Read the model definition and answer for the solid it produces. Units are mm, in the model's axes. Face numbers are marked on the shaded views. A direction names the side the tool comes from. Coordinates: 2 decimals unless noted, no trailing zeros. Write each loop counter-clockwise with the first axis right and the second up, starting at its lowest first coordinate (ties: lowest second). Pieces come first, ordered by that corner, then holes.
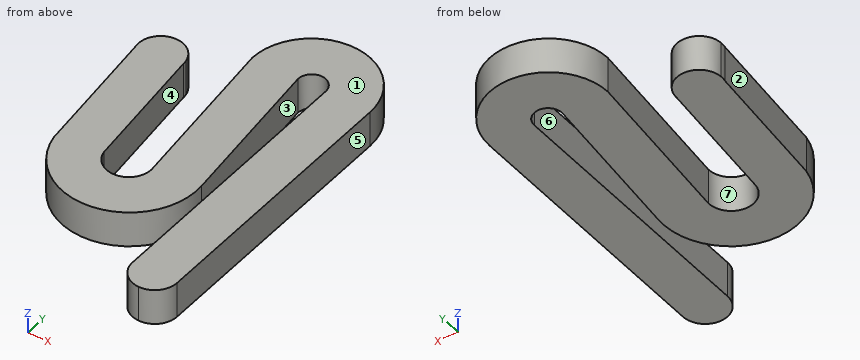
from build123d import *

# Parameters (mm, degrees)
F1_DEPTH = 5.08


with BuildPart() as f1:
    # F0 (on Top) → F1 (new body)
    with BuildSketch(Plane.XY):
        with BuildLine():
            Line((0.549417, 29.093022), (0.549417, -9.006978))
            ThreePointArc((0.549417, -9.006978), (1.479353, -11.252042), (3.724417, -12.181978))
            ThreePointArc((3.724417, -12.181978), (5.969481, -11.252042), (6.899417, -9.006978))
            Line((6.899417, -9.006978), (6.899417, 29.093022))
            ThreePointArc((6.899417, 29.093022), (-1.509537, 37.488393), (-9.891303, 29.065877))
            Line((-9.891303, 29.065877), (-7.490417, 5.875438))
            ThreePointArc((-7.490417, 5.875438), (-10.365969, 2.64314), (-13.81069, 5.260477))
            Line((-13.81069, 5.260477), (-15.701351, 23.522593))
            Line((-15.701351, 23.522593), (-15.762292, 24.111232))
            ThreePointArc((-15.762292, 24.111232), (-19.158057, 26.675151), (-22.092695, 23.594112))
            Line((-22.092695, 23.594112), (-22.003429, 22.731883))
            Line((-22.003429, 22.731883), (-20.061784, 3.977299))
            ThreePointArc((-20.061784, 3.977299), (-9.191107, -3.629406), (-1.073799, 6.865493))
            Line((-1.073799, 6.865493), (-3.372185, 29.065877))
            ThreePointArc((-3.372185, 29.065877), (-1.425051, 31.05387), (0.549417, 29.093022))
        make_face()
        with BuildLine():
            ThreePointArc((-22.092695, 23.594112), (-22.077424, 23.159958), (-22.003429, 22.731883))
            Line((-22.003429, 22.731883), (-22.092695, 23.594112))
        make_face()
        with BuildLine():
            ThreePointArc((-15.701351, 23.522593), (-15.718171, 23.818326), (-15.762292, 24.111232))
            Line((-15.762292, 24.111232), (-15.701351, 23.522593))
        make_face()
    extrude(amount=F1_DEPTH)


solid = f1.part
Item 1: For the marked faces 5, 6 and 7, determine the directions among +Z, -Z, +X, -X, +Y, -Y from which every point of the face is accessible in a straight line to the end or side of a thin tool.
Item 2: The part is cut by section B-B (x = -2.5). Give the vertices of the cut face in (y, z).
Item 3: Determine the mould class of the marked faces 1, 2, 3 and 4 for opening direction Y: +Y half, -Y half, draft (parallel to the pull), parting line (faces both ways), or undercut.
Item 4: Given pin 1 (1 mm diameter, centred on x = -4, z = 3, fed in from +Y), flat-ended and moving along its own axis, determine where the tip first touches the part or whether it passes through.
Item 5: The part is cut by section D-D (y = 13.5). Give the vertices of the cut face in (x, z).
Item 6: Find the intervals of material crossed by probe 1 along X at (y, z) = (29, 3.6); probe 2 along X at (y, z) = (4, 1.4); probe 3 along X at (y, z) = (15.5, 2.55), in increasing order.
Item 7: The part is cut by section C-C (y = -3). Give the vertices of the cut face in (x, z).
Answer:
1. face 5: +Z, -Z, +X, +Y, -Y
1. face 6: +Z, -Z, -Y
1. face 7: +Z, -Z
2. outline: (0.75, 0) - (20.64, 0) - (20.64, 5.08) - (0.75, 5.08) - close; (30.72, 0) - (37.43, 0) - (37.43, 5.08) - (30.72, 5.08) - close
3. face 1: draft
3. face 2: -Y half
3. face 3: undercut
3. face 4: +Y half
4. pin 1: stops at y = 37.25
5. outline: (-21.05, 0) - (-14.66, 0) - (-14.66, 5.08) - (-21.05, 5.08) - close; (-8.28, 0) - (-1.76, 0) - (-1.76, 5.08) - (-8.28, 5.08) - close; (0.55, 0) - (6.9, 0) - (6.9, 5.08) - (0.55, 5.08) - close
6. probe 1: x = -9.88 to -3.37, 0.55 to 6.9
6. probe 2: x = -20.06 to -13.29, -8.06 to -1.21, 0.55 to 6.9
6. probe 3: x = -21.25 to -14.87, -8.49 to -1.97, 0.55 to 6.9
7. outline: (-14.33, 0) - (-6.94, 0) - (-6.94, 5.08) - (-14.33, 5.08) - close; (0.55, 0) - (6.9, 0) - (6.9, 5.08) - (0.55, 5.08) - close
